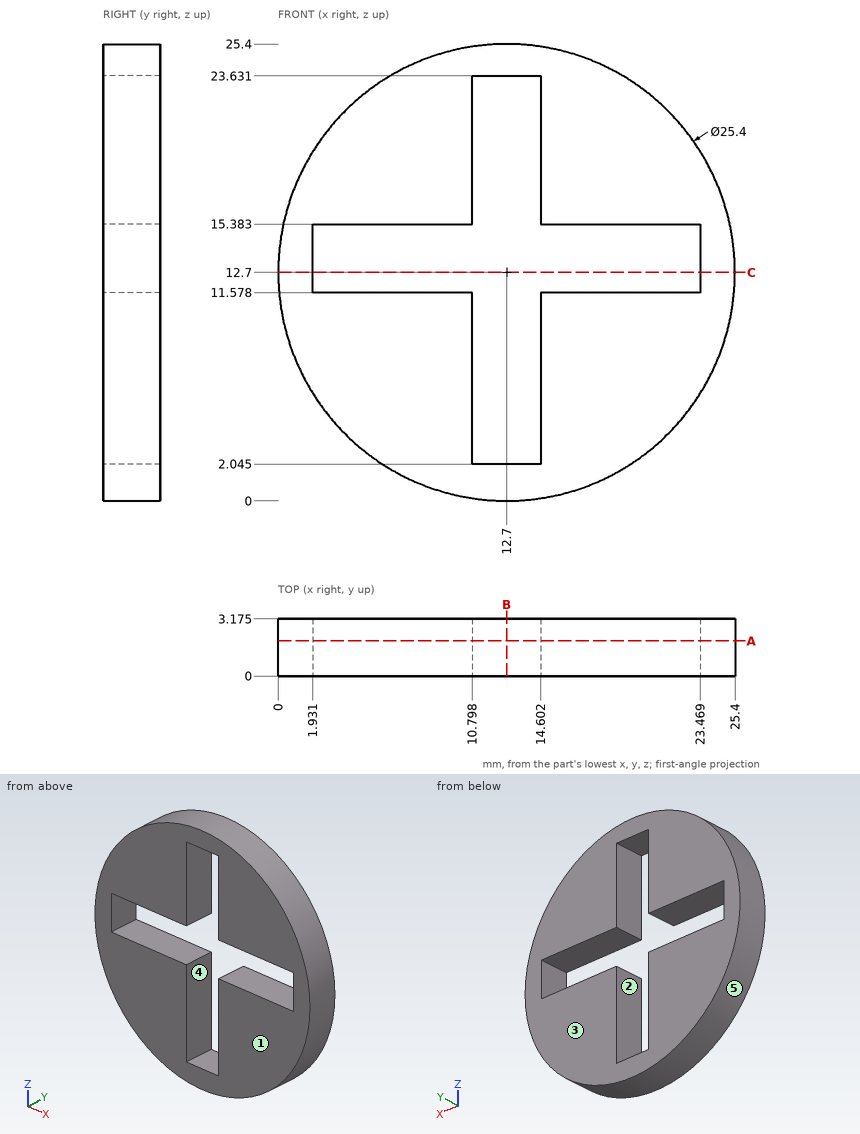
Design review of the part shown in the three views and the two pictorial views. Dimensions are in mm from the part's minimum x, y and z. A direction names the side the tool comes from. Round coordinates to 2 decimals unless told otherwise and drop trailing zeros. Loops run counter-clockwise (first coordinate to the right, second up) from the corner with the lowest first, then second, coordinate; pieces in that order, holes last. Notation, with made-up numbers: (73, 33.5) -> (121, 33.5) arc R29 cw to (121, 53.5) -> close; hole circle Ø6 at (-15, 11). An arc over 180 degrees is marked (long way). Return JSON: item names as keys, results as strings.
(1) For the marked faces 1 and 2, list the 3-axis set-ups (+Z, -Z, +X, -X, +Y, -Y) from which the entire face can be reached by the end or side of a thin tool; tool diameter is ignored.
Solved:
{"face 1": "+Z, -Z, +X, -X, -Y", "face 2": "+Y, -Y"}
(2) Add section C-C on z = 12.7. Write out the cut boundary in (x, y) (1 decimal).
Solved:
{"outline": "(0, 0) -> (1.9, 0) -> (1.9, 3.2) -> (0, 3.2) -> close; (23.5, 0) -> (25.4, 0) -> (25.4, 3.2) -> (23.5, 3.2) -> close"}
(3) For line 1 (Z direction, x = 12.5, y = 2.5) (1 decimal); line 2 (Z direction, x = 19.25, y = 1.5) (1 decimal); line 3 (X direction, y = 2.8, z = 11.25), list the stretches that pass through material, from the lowest coordinate up.
Solved:
{"line 1": "0 to 2, 23.6 to 25.4", "line 2": "1.8 to 11.6, 15.4 to 23.6", "line 3": "0.08 to 10.8, 14.6 to 25.32"}
(4) For pin 1 (1.6 mm diameter, centred on x = 19.5, y = 2, fed in from -Z); pin 2 (1.6 mm diameter, centred on y = 2, z = 20.5, fed in from +X); pin 3 (1 mm diameter, centred on y = 1.5, z = 14, fed in from +X) (1 decimal), all flat-tipped, find the tip position at first contact; note any pin that passes through.
Solved:
{"pin 1": "z = 1.51", "pin 2": "x = 23.3", "pin 3": "x = 25.4"}
(5) Add section B-B on x = 12.7. Write out the cut boundary in (y, z) (1 decimal), plus the area to 3 significant figures.
Solved:
{"outline": "(0, 0) -> (3.2, 0) -> (3.2, 2) -> (0, 2) -> close; (0, 23.6) -> (3.2, 23.6) -> (3.2, 25.4) -> (0, 25.4) -> close", "area": "12.1 mm2"}
(6) Add section A-A on y = 1.95. Write out the cut boundary in (x, z) (1 decimal), plus the area to 3 significant figures.
Solved:
{"outline": "circle Ø25.4 at (12.7, 12.7); hole (1.9, 11.6) -> (10.8, 11.6) -> (10.8, 2) -> (14.6, 2) -> (14.6, 11.6) -> (23.5, 11.6) -> (23.5, 15.4) -> (14.6, 15.4) -> (14.6, 23.6) -> (10.8, 23.6) -> (10.8, 15.4) -> (1.9, 15.4) -> close", "area": "357 mm2"}
(7) The part is to be moulded in two halves that separate along Z. For the marked faces 3, 4 and 5, say which applies: released by +Z, released by -Z, zero draft, split by the parting line, or undercut.
Solved:
{"face 3": "zero draft", "face 4": "undercut", "face 5": "split by the parting line"}
